Drawing for the job (mm, zero at the part's lowest x, y, z). Round coordinates to 2 decimals unless told otherwise and drop trailing zeros. Write each loop counter-clockwise with the first axis right and the second up, starting at its lowest first coordinate (ties: lowest second). Pieces come first, ordered by that corner, then holes. Notation, with made-up numbers: M 61.25,68.25 L 78.25,68.25 A14 ccw 78.25,88.25 Z; hole C 59,-13.75 d7. An arc over 180 degrees is marked long. Use a Markdown table: item, result.
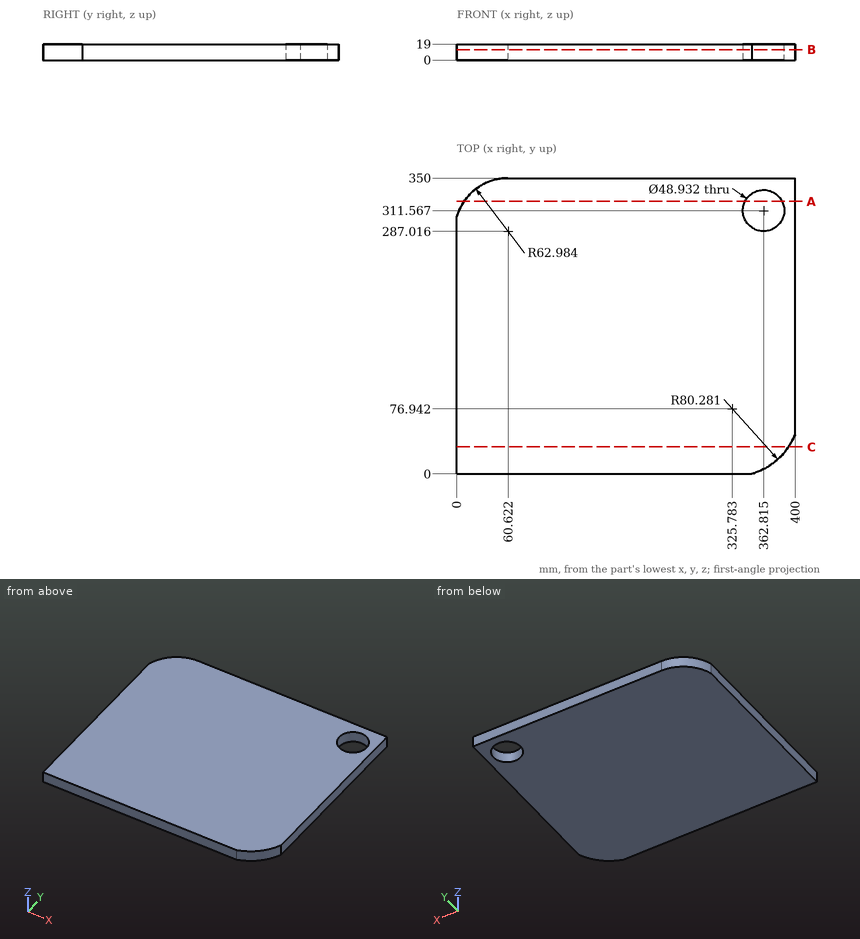
Q1. Cut at B-B on z = 12.25. Give the cut face in (x, y) (1 decimal), and give its area (3 significant figures).
Response values:
| item | result |
|---|---|
| outline | M 0,0 L 348.7,0 A80.3 ccw 400,46.3 L 400,350 L 60.4,350 A63 ccw 0,304.1 Z; hole C 362.8,311.6 d48.9 |
| area | 137,000 mm2 |
Q2. Drill centre line: L1, parallel to Y at x = 380.5, z = 11.5 (1 decimal). Where is it in solid material? Low to high.
Response values:
| item | result |
|---|---|
| L1 | y = 18.2 to 294.7, 328.5 to 350 |
Q3. Cut at C-C on y = 32. Give the cut face in (x, z).
Response values:
| item | result |
|---|---|
| outline | M 0,0 L 392.31,0 L 392.31,19 L 0,19 Z |
Q4. Cut at A-A on y = 322.5. Give the cut face in (x, z) (1 decimal).
Response values:
| item | result |
|---|---|
| outline | M 8.6,0 L 340.9,0 L 340.9,19 L 8.6,19 Z; M 384.7,0 L 400,0 L 400,19 L 384.7,19 Z |
